from build123d import *

# Parameters (mm, degrees)
SKETCH_1_R      = 4.5
EXTRUDE_1_DEPTH = 10
SKETCH_2_R      = 11
EXTRUDE_2_DEPTH = 25
FILLET_1_R      = 2
CHAMFER_1_SIZE  = 1


with BuildPart() as part:
    # Эскиз1 → Бобышка-Вытянуть1 (new body)
    with BuildSketch(Plane(origin=(0, 0, 0), x_dir=(1, 0, 0), z_dir=(0, 1, 0))):
        with BuildLine():
            Line((-25.608695652, 9.65374057), (-4.173913043, 15.445984912))
            ThreePointArc((-4.173913043, 15.445984912), (0, 16), (4.173913043, 15.445984912))
            Line((4.173913043, 15.445984912), (25.608695652, 9.65374057))
            ThreePointArc((25.608695652, 9.65374057), (33, 0), (25.608695652, -9.65374057))
            Line((25.608695652, -9.65374057), (4.173913043, -15.445984912))
            ThreePointArc((4.173913043, -15.445984912), (0, -16), (-4.173913043, -15.445984912))
            Line((-4.173913043, -15.445984912), (-25.608695652, -9.65374057))
            ThreePointArc((-25.608695652, -9.65374057), (-33, 0), (-25.608695652, 9.65374057))
        make_face()
        with Locations(Location((-23, 0, 0), (0, 0, 270))):
            Circle(SKETCH_1_R, mode=Mode.SUBTRACT)
        with Locations(Location((23, 0, 0), (0, 0, 90))):
            Circle(SKETCH_1_R, mode=Mode.SUBTRACT)
    extrude(amount=-EXTRUDE_1_DEPTH)

    # Эскиз2 → Бобышка-Вытянуть2 (add)
    with BuildSketch(Plane(origin=(0, 0, 0), x_dir=(1, 0, 0), z_dir=(0, 1, 0))):
        with Locations(Location((0, 0, 0), (0, 0, 270))):
            Circle(SKETCH_2_R)
    extrude(amount=-EXTRUDE_2_DEPTH)

    # Эскиз3 → Вырез-Повернуть1 (revolve, cut)
    with BuildSketch(Plane.XY, mode=Mode.PRIVATE) as cut_revolve_1_sk:
        with BuildLine():
            Line((0, 0), (-10, 0))
            Line((-10, 0), (-8.122654092, -13.141421356))
            ThreePointArc((-8.122654092, -13.141421356), (-7.78790634, -13.755453955), (-7.132704598, -14))
            Line((-7.132704598, -14), (-6, -14))
            Line((-6, -14), (-6, -25))
            Line((-6, -25), (0, -25))
            Line((0, -25), (0, 0))
        make_face()
    revolve(cut_revolve_1_sk.sketch.rotate(Axis((0, 4.006279318, 0), (0, -1, 0)), 270), axis=Axis((0, 4.006279318, 0), (0, -1, 0)), mode=Mode.SUBTRACT)

    # Скругление1
    fillet_1_edges = [part.edges().sort_by_distance(p)[0] for p in [
        (0, -10, -11),
    ]]
    fillet(fillet_1_edges, radius=FILLET_1_R)

    # Фаска1
    chamfer_1_edges = [part.edges().sort_by_distance(p)[0] for p in [
        (0, -25, -11),
    ]]
    chamfer(chamfer_1_edges, length=CHAMFER_1_SIZE)


solid = part.part
Read the model definition and answer for the solid it produces. Units are mm, in the model's axes. A direction names the side the tool comes from. Round coordinates to 2 decimals unless told otherwise and drop trailing zeros. Write each loop counter-clockwise with the first axis right and the second up, starting at its lowest first coordinate (ties: lowest second). Pieces come first, ordered by that corner, then holes. Notation, with made-up numbers: (-29, 58) - (-3, 58) arc R8 cw to (-3, 73) - close; hole circle Ø11 at (-29.75, 88). An arc over 180 degrees is marked (long way). Use a Markdown table: item, result.
(1) Which of the six approach directions +Z, -Z, +X, -X, +Y, -Y give full straight-line access (tool end or side, diameter ignored) to faces 1 (the flat face through (-6, -14, -2)), 2 (the cylindrical face through (-10.74, -17.92, -2.38)), 3 (the cylindrical face through (-33, -5, 0))?
Reported:
| item | result |
|---|---|
| face 1 | +Y |
| face 2 | -Y |
| face 3 | -X, +Y, -Y |
(2) The part is cut by section A-A (z = 0). State how many separate pieces and enclosed holes the cut face has, then the cut area to 3 significant figures.
Reported:
| item | result |
|---|---|
| separate pieces | 4 |
| enclosed holes | 0 |
| area | 427 mm2 |
(3) The part is cut by section C-C (y = -2.75). Write down the section's boundary in (x, z).
Reported:
| item | result |
|---|---|
| outline | (-25.61, -9.65) - (-4.17, -15.45) arc R16 ccw to (4.17, -15.45) - (25.61, -9.65) arc R10 ccw to (25.61, 9.65) - (4.17, 15.45) arc R16 ccw to (-4.17, 15.45) - (-25.61, 9.65) arc R10 ccw to start; hole circle Ø9 at (-23, 0); hole circle Ø19.21 at (0, 0); hole circle Ø9 at (23, 0) |
(4) Straight lines are drawn through the part: line 1 along X through (y, z) = (-15.75, 0); line 2 along Y through (x, z) = (21, 8); line 3 along Z through (x, y) = (-2, -8). For each, find the intervals that lie inside material, in ascending order. Write a range as [from, to].
Reported:
| item | result |
|---|---|
| line 1 | [-11, -6], [6, 11] |
| line 2 | [-10, 0] |
| line 3 | [-15.87, -8.63], [8.63, 15.87] |
(5) The part is cut by section D-D (x = -19.5). Write down the section's boundary in (y, z), then the cut area to 3 significant figures.
Reported:
| item | result |
|---|---|
| outline | (-10, -11.3) - (0, -11.3) - (0, -2.83) - (-10, -2.83) - close; (-10, 2.83) - (0, 2.83) - (0, 11.3) - (-10, 11.3) - close |
| area | 170 mm2 |
(6) Each of these flat-tipped pins is pushed along its axis until it touches: pin 1 Ø1 at (x, y) = (8.5, -3.5) entering from -Z; pin 2 Ø1 at (x, z) = (-16, -4.5) entering from -Y; pin 3 Ø12 at (y, z) = (-7, -6.5) entering from +X. Where does it stop, or does it pass through?
Reported:
| item | result |
|---|---|
| pin 1 | z = -14.41 |
| pin 2 | y = -10 |
| pin 3 | x = 32.99 |
(7) The part is cut by section B-B (x = 0). Write down the section's boundary in (y, z), then the cut area to 3 significant figures.
Reported:
| item | result |
|---|---|
| outline | (-25, -10) - (-24, -11) - (-12, -11) arc R2 cw to (-10, -13) - (-10, -16) - (0, -16) - (0, -10) - (-13.14, -8.12) arc R1 cw to (-14, -7.13) - (-14, -6) - (-25, -6) - close; (-25, 6) - (-14, 6) - (-14, 7.13) arc R1 cw to (-13.14, 8.12) - (0, 10) - (0, 16) - (-10, 16) - (-10, 13) arc R2 cw to (-12, 11) - (-24, 11) - (-25, 10) - close |
| area | 267 mm2 |
(8) The mould has two halves that part along Z. Classify faces 4 (the cylindrical face through (33, -5, 0)), 5 (the cylindrical face through (0, -5, 16)), 6 (the conical face through (-2.66, -8.12, 8.43)), 7 (the flat face through (-7, -25, 0)): released by +Z, released by -Z, zero draft, split by the parting line, or undercut.
Reported:
| item | result |
|---|---|
| face 4 | split by the parting line |
| face 5 | released by +Z |
| face 6 | undercut |
| face 7 | zero draft |
